Design review of the part built by this model. Coordinates are the model's own, in mm. Face numbers are marked on the shaded views. A direction names the side the tool comes from. Round coordinates to 2 decimals unless told otherwise and drop trailing zeros. Order: outer loops, then holes, each group sorted by start corner. A loop starts at its lowest first (then second) coordinate and runs counter-clockwise, first axis right, second up. Notation, with made-up numbers: M -19.75,60 L 32.25,60 A17 ccw 32.25,83 Z; hole C 55.25,-34 d7. An arc over 180 degrees is marked long. Use a Markdown table: item, result. Add a question column.
(1) The part is to be moulded in two halves that separate along X. For the marked faces 4, 5, 6 and 7, say which applies: released by +X, released by -X, zero draft, split by the parting line, or undercut.
(2) Take a section at B-B (z = -8.5). Write out the cut boundary in (x, y).
(3) To check wall thickness, follow probe 1 along Z at (x, y) = (-4, 0); probe 2 along X at (y, z) = (1, 3.25); probe 3 along X at (y, z) = (-0.5, -5). State the ranges of each line that lie inside material, in increasing order. Write a range as from..to.
(4) For pin 1 (0.8 mm diameter, centred on x = -32, y = 22, fed in from -Z); pin 2 (2 mm diameter, centred on x = -31.5, z = -4, fed in from -Y); pin 3 (8.5 mm diameter, centred on x = -35, y = 0, fed in from +Z); pin 4 (4.5 mm diameter, centred on x = -18, z = -7.5, fed in from +Y), all flat-tipped, find the tip position at first contact; note any pin that passes through.
(5) Take a section at C-C (y = 0). Write out the cut boundary in (x, z).
(6) Take a section at D-D (z = -0.4). Write out the cut boundary in (x, y), then the cut area to 3 significant figures.
(7) Machinability: for the marked faces 1, 2 and 3, which of the approach directions +Z, -Z, +X, -X, +Y, -Y give a long, thin tool a straight path to every point of the face, cutting with its end or side? Answer none if there is none.
(8) Take a section at A-A (x = -35). Write out the cut boundary in (y, z).
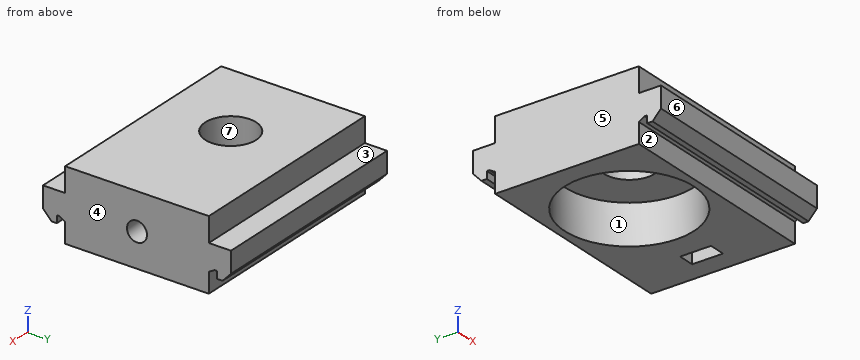
Autodesk Fusion 360 part; units mm, degrees
sketch "Main Profile" plane through (0, 0, 0) normal (1, 0, 0) x (0, 1, 0)
  line L0 (-19.75, -9.75) -> (19.75, -9.75)
  line L1 (19.75, -9.75) -> (19.75, 9.75)
  line L2 (19.75, 9.75) -> (-19.75, 9.75)
  line L3 (-19.75, 9.75) -> (-19.75, -9.75)
  line L4 (-19.75, -9.75) -> (19.75, 9.75) construction
  line L5 (19.75, -9.75) -> (-19.75, 9.75) construction
  line L6 (-19.75, 3) -> (-25.85, 3)
  line L7 (-25.85, 3) -> (-25.85, -2.8)
  line L8 (-25.85, -2.8) -> (-23.5187, -5.3)
  line L9 (-23.5187, -5.3) -> (-22.05, -5.3)
  line L10 (-22.05, -5.3) -> (-22.05, -3.3)
  line L11 (-22.05, -3.3) -> (-21.35, -3.3)
  line L12 (-21.35, -3.3) -> (-19.75, -4.2238)
  line L13 (0, 9.75) -> (0, -9.75) construction
  line L14 (19.75, 3) -> (25.85, 3)
  line L15 (25.85, 3) -> (25.85, -2.8)
  line L16 (25.85, -2.8) -> (23.5187, -5.3)
  line L17 (23.5187, -5.3) -> (22.05, -5.3)
  line L18 (22.05, -5.3) -> (22.05, -3.3)
  line L19 (22.05, -3.3) -> (21.35, -3.3)
  line L20 (21.35, -3.3) -> (19.75, -4.2238)
  circle A0 centre (0, -0.4) radius 2.75
  dimension "d1" = 39.5
  dimension "d2" = 19.5
  dimension "d3" = 6.1
  dimension "d4" = 6.75
  dimension "d5" = 8.3
  dimension "d6" = 43
  dimension "d7" = 2.5
  dimension "d8" = 120
  dimension "d9" = 3.8
  dimension "d10" = 2
  dimension "d11" = 1.6
  dimension "d12" = 5.5
  dimension "d13" = 0.4
extrude "Extrude1" add sketch "Main Profile" against normal blind 58.25 contours L0 L1 L2 L3 | L3 L6 L7 L8 L9 L10 L11 L12 | L1 L14 L15 L16 L17 L18 L19 L20 | A0
sketch "Side" plane through (0, 0, -9.75) normal (0, 0, -1) x (1, 0, 0)
  line L0 (0, -19.75) -> (0, 19.75)
  line L1 (0, 19.75) -> (-58.25, 19.75)
  line L2 (-58.25, 19.75) -> (-58.25, -19.75)
  line L3 (-58.25, -19.75) -> (0, -19.75)
  circle A0 centre (-35, 0) radius 17.75
  circle A1 centre (-35, 0) radius 7
  line L4 (-10.25, -4.25) -> (-5.75, -4.25)
  line L5 (-5.75, -4.25) -> (-5.75, 4.25)
  line L6 (-5.75, 4.25) -> (-10.25, 4.25)
  line L7 (-10.25, 4.25) -> (-10.25, -4.25)
  line L8 (-10.25, -4.25) -> (-5.75, 4.25) construction
  line L9 (-5.75, -4.25) -> (-10.25, 4.25) construction
  point P0 (-8, 0)
  dimension "d16" = 35.5
  dimension "d17" = 35
  dimension "d18" = 14
  dimension "d19" = 8.5
  dimension "d20" = 4.5
  dimension "d21" = 5.75
extrude "Extrude2" cut sketch "Side" against normal blind 13.5 contours L4 L5 L6 L7
extrude "Extrude3" cut sketch "Side" against normal blind 40 contours A1
extrude "Extrude4" cut sketch "Side" against normal blind 10.85 contours A0
extrude "Extrude5" cut sketch "Main Profile" against normal blind 15.75 contours A0
extrude "Extrude6" cut 1 faces at (-20.8994, 0.8818, 1.1) along direction (0, 0, 1) blind 0.15
Verdict:
| question | item | result |
|---|---|---|
| 1 | face 4 | released by +X |
| 1 | face 5 | released by -X |
| 1 | face 6 | zero draft |
| 1 | face 7 | undercut |
| 2 | outline | M -58.25,-19.75 L 0,-19.75 L 0,19.75 L -58.25,19.75 Z; hole C -35,0 d35.5; hole M -10.25,-4.25 L -5.75,-4.25 L -5.75,4.25 L -10.25,4.25 Z |
| 3 | probe 1 | z = -9.75..-3.15, 2.35..9.75 |
| 3 | probe 2 | x = -58.25..-41.93, -28.07..-10.25, -5.75..0 |
| 3 | probe 3 | x = -58.25..-52.74, -17.26..-10.25, -5.75..0 |
| 4 | pin 1 | stops at z = -5.3 |
| 4 | pin 2 | stops at y = -25.66 |
| 4 | pin 3 | passes through |
| 4 | pin 4 | stops at y = 23.57 |
| 5 | outline | M -58.25,-9.75 L -52.75,-9.75 L -52.75,1.25 L -42,1.25 L -42,9.75 L -58.25,9.75 Z; M -28,1.25 L -17.25,1.25 L -17.25,-9.75 L -10.25,-9.75 L -10.25,-3.15 L -15.75,-3.15 L -15.75,2.35 L -10.25,2.35 L -10.25,3.75 L -5.75,3.75 L -5.75,2.35 L 0,2.35 L 0,9.75 L -28,9.75 Z; M -5.75,-9.75 L 0,-9.75 L 0,-3.15 L -5.75,-3.15 Z |
| 6 | outline | M -58.25,-25.85 L 0,-25.85 L 0,-2.75 L -5.75,-2.75 L -5.75,-4.25 L -10.25,-4.25 L -10.25,-2.75 L -15.75,-2.75 L -15.75,2.75 L -10.25,2.75 L -10.25,4.25 L -5.75,4.25 L -5.75,2.75 L 0,2.75 L 0,25.85 L -58.25,25.85 Z; hole C -35,0 d35.5 |
| 6 | area | 1,920 mm^2 |
| 7 | face 1 | -Z |
| 7 | face 2 | -Z, +X, -X |
| 7 | face 3 | +Z, +X, -X, +Y |
| 8 | outline | M -25.85,-2.8 L -23.52,-5.3 L -22.05,-5.3 L -22.05,-3.3 L -21.35,-3.3 L -19.75,-4.22 L -19.75,-9.75 L -17.75,-9.75 L -17.75,1.25 L -7,1.25 L -7,9.75 L -19.75,9.75 L -19.75,3 L -25.85,3 Z; M 7,1.25 L 17.75,1.25 L 17.75,-9.75 L 19.75,-9.75 L 19.75,-4.22 L 21.35,-3.3 L 22.05,-3.3 L 22.05,-5.3 L 23.52,-5.3 L 25.85,-2.8 L 25.85,3 L 19.75,3 L 19.75,9.75 L 7,9.75 Z |
